from build123d import *

# Parameters (mm, degrees)
F0_W     = 127
F0_H     = 127
F1_DEPTH = 38.1
F2_R     = 21.59
F4_DEPTH = 30.48
F7_DEPTH = 1270


with BuildPart() as f1:
    # F0 (on Top) → F1 (new body)
    with BuildSketch(Plane.XY):
        Rectangle(F0_W, F0_H)
    extrude(amount=F1_DEPTH)

    # F2 (on face) → F4 (join)
    with BuildSketch(Plane.XY.offset(38.1)):
        Circle(F2_R)
    extrude(amount=F4_DEPTH)

    # F6 (on offset) → F7 (cut)
    with BuildSketch(Plane.XZ.offset(25.4)):
        Polygon((21.590049, 68.58), (-21.590006, 68.58), (21.590049, 43.18), align=None)
    extrude(amount=-F7_DEPTH, mode=Mode.SUBTRACT)


solid = f1.part
Could you check a few things on this model? Use its own coordinates, in mm. A direction names the side the tool comes from. Give positions to 0.01 mm unless a question says otherwise; leave off trailing zeros. Order: outer loops, then holes, each group sorted by start corner. A loop starts at its lowest first (then second) coordinate and runs counter-clockwise, first axis right, second up.
1. For faces 1 (the cylindrical face through (-21.57, 0.95, 49.94)), 2 (the flat face through (-1, 63.5, 19)), which set-ups out of +Z, -Z, +X, -X, +Y, -Y let a thin tool reach every point of the face, with its end or its side?
2. We'd pull the mould along Z, two halves only. Please class faces 3 (the flat face through (-1, 1, 0)), 4 (the flat face through (27, 1, 38.1)), 5 (the flat face through (-63.5, -1, 19)): pulls with the +Z half, pulls with the -Z half, needs draft (parallel to the pull), parting line crosses it, or undercut.
3. Suppose I cut it at B-B (x = 1.5). List the corners of the cut face in (y, z) for me, plus the area to 3 significant figures.
4. Will these pins go through, and if not, where does the flat tip stop? P1, Ø1.5, axis at x = 19, y = 46.5, coming from the +Z side; P2, Ø10, axis at y = 15, z = 52, coming from the +X side.
5. Suppose I cut it at C-C (x = -31.5). List the corners of the cut face in (y, z) for me, plus the area to 3 significant figures.
6. I need wall thicknesses on L1, parallel to Z at x = 53, y = 45.5; L2, parallel to Z at x = -5, y = -18.5. Which ranges of each line are inside material? Lowest first, please.
7. Suppose I cut it at A-A (y = 0). List the corners of the cut face in (x, z) for me, plus the area to 3 significant figures.
Solved:
1. face 1: +Z
1. face 2: +Z, -Z, +X, -X, +Y
2. face 3: pulls with the -Z half
2. face 4: pulls with the +Z half
2. face 5: needs draft
3. outline: (-63.5, 0) - (63.5, 0) - (63.5, 38.1) - (21.54, 38.1) - (21.54, 55) - (-21.54, 55) - (-21.54, 38.1) - (-63.5, 38.1) - close
3. area: 5,570 mm2
4. P1: stops at z = 38.1
4. P2: stops at x = 15.1
5. outline: (-63.5, 0) - (63.5, 0) - (63.5, 38.1) - (-63.5, 38.1) - close
5. area: 4,840 mm2
6. L1: z = 0 to 38.1
6. L2: z = 0 to 58.82
7. outline: (-63.5, 0) - (63.5, 0) - (63.5, 38.1) - (21.59, 38.1) - (21.59, 43.18) - (-21.59, 68.58) - (-21.59, 38.1) - (-63.5, 38.1) - close
7. area: 5,610 mm2
